from build123d import *

# Parameters (mm, degrees)
SKETCH1_R           = 7
SKETCH1_R_2         = 5.5
BOSS_EXTRUDE1_DEPTH = 7
SKETCH2_R           = 7
SKETCH2_R_2         = 4
BOSS_EXTRUDE2_DEPTH = 7
BOSS_EXTRUDE3_DEPTH = 4.5
CUT_EXTRUDE2_DEPTH  = 2


with BuildPart() as part:
    # Sketch1 → Boss-Extrude1 (new body, symmetric)
    with BuildSketch(Plane.XY):
        Circle(SKETCH1_R)
        Circle(SKETCH1_R_2, mode=Mode.SUBTRACT)
    extrude(amount=BOSS_EXTRUDE1_DEPTH, both=True)



with BuildPart() as body_2:
    # Sketch2 → Boss-Extrude2 (new body, symmetric)
    with BuildSketch(Plane.XY):
        with Locations((0, 80)):
            Circle(SKETCH2_R)
        with Locations((0, 80)):
            Circle(SKETCH2_R_2, mode=Mode.SUBTRACT)
    extrude(amount=BOSS_EXTRUDE2_DEPTH, both=True)


with BuildPart() as part_1:
    add(part.part)

    add(body_2.part)  # Boss-Extrude3 merges body 2
    # Sketch3 → Boss-Extrude3 (add, symmetric)
    with BuildSketch(Plane.XY):
        with BuildLine():
            Line((-5.25, 75.369935206), (-5.25, 4.630064794))
            ThreePointArc((-5.25, 4.630064794), (0, 7), (5.25, 4.630064794))
            Line((5.25, 4.630064794), (5.25, 75.369935206))
            ThreePointArc((5.25, 75.369935206), (0, 73), (-5.25, 75.369935206))
        make_face()
    extrude(amount=BOSS_EXTRUDE3_DEPTH, both=True)

    # Sketch4 → Cut-Extrude2 (cut)
    with BuildSketch(Plane.XY.offset(4.5)):
        with BuildLine():
            ThreePointArc((-3, 67.154767421), (-2.650443636, 67.914321947), (-1.846153846, 68.142862235))
            ThreePointArc((-1.846153846, 68.142862235), (0, 68), (1.846153846, 68.142862235))
            ThreePointArc((1.846153846, 68.142862235), (2.650443636, 67.914321947), (3, 67.154767421))
            Line((3, 67.154767421), (3, 12.845232579))
            ThreePointArc((3, 12.845232579), (2.650443636, 12.085678053), (1.846153846, 11.857137765))
            ThreePointArc((1.846153846, 11.857137765), (0, 12), (-1.846153846, 11.857137765))
            ThreePointArc((-1.846153846, 11.857137765), (-2.650443636, 12.085678053), (-3, 12.845232579))
            Line((-3, 12.845232579), (-3, 67.154767421))
        make_face()
    cut_extrude2 = extrude(amount=-CUT_EXTRUDE2_DEPTH, mode=Mode.SUBTRACT)

    # Mirror1: Cut-Extrude2 across plane
    add(cut_extrude2.mirror(Plane.XY), mode=Mode.SUBTRACT)


solid = part_1.part
The listing builds one solid part. Answer for the finished solid, in the listing's coordinates (mm). A direction names the side the tool comes from. Round coordinates to 2 decimals unless told otherwise and drop trailing zeros. Order: outer loops, then holes, each group sorted by start corner. A loop starts at its lowest first (then second) coordinate and runs counter-clockwise, first axis right, second up. Notation, with made-up numbers: (-27.75, -3) - (-14.75, -3) arc R21 ccw to (-14.75, 31) - close; hole circle Ø8 at (54.5, -31.75). An arc over 180 degrees is marked (long way). Write item = value, one per line. Start each with the question number.
1) Section A-A, the plane x = 0 is taken. Write down the section's boundary in (y, z).
2) Given pin 1 (3 mm diameter, centred on x = 2.5, y = 34.5, fed in from +Z); pin 2 (2 mm diameter, centred on x = -1.5, y = 47, fed in from +Z); pin 3 (0.6 mm diameter, centred on y = 44.5, z = 3.5, fed in from +X), each flat-ended and moving along its own axis, determine where each tip first touches the part or whether it passes through.
3) Section D-D, the plane y = 27 is taken. Write down the section's boundary in (x, z), plus the area to 3 significant figures.
4) Straight lines are drawn through the part: L1, parallel to Y at x = 0, z = -2; L2, parallel to X at y = 25, z = -2.75; L3, parallel to Y at x = 1.25, z = 3.5. For each, find the intervals that lie inside material, in ascending order.
5) For faces 1 (the cylindrical face through (0, 68, 4)), 2 (the flat face through (5.25, 40, 0)), 3 (the cylindrical face through (0, 68, -4)), 4 (the flat face through (-5.25, 40, 0)), determine the directions among +Z, -Z, +X, -X, +Y, -Y from which every point of the face is accessible in a straight line to the end or side of a thin tool.
6) Section B-B, the plane y = 80 is taken. Write down the section's boundary in (x, z), plus the area to 3 significant figures.
7) Section C-C, the plane z = -5.5 is taken. Write down the section's boundary in (x, y), plus the area to 3 significant figures.
Results list:
q1.outline = (-7, -7) - (-5.5, -7) - (-5.5, 7) - (-7, 7) - close; (5.5, -7) - (7, -7) - (7, -4.5) - (12, -4.5) - (12, -2.5) - (68, -2.5) - (68, -4.5) - (73, -4.5) - (73, -7) - (76, -7) - (76, 7) - (73, 7) - (73, 4.5) - (68, 4.5) - (68, 2.5) - (12, 2.5) - (12, 4.5) - (7, 4.5) - (7, 7) - (5.5, 7) - close; (84, -7) - (87, -7) - (87, 7) - (84, 7) - close
q2.pin_1 = 4.5
q2.pin_2 = 2.5
q2.pin_3 = 5.25
q3.outline = (-5.25, -4.5) - (-3, -4.5) - (-3, -2.5) - (3, -2.5) - (3, -4.5) - (5.25, -4.5) - (5.25, 4.5) - (3, 4.5) - (3, 2.5) - (-3, 2.5) - (-3, 4.5) - (-5.25, 4.5) - close
q3.area = 70.5 mm^2
q4.L1 = -7 to -5.5, 5.5 to 76, 84 to 87
q4.L2 = -5.25 to -3, 3 to 5.25
q4.L3 = -6.89 to -5.36, 5.36 to 11.93, 68.07 to 76.2, 83.8 to 86.89
q5.face_1 = +Z
q5.face_2 = +Z, -Z, +X
q5.face_3 = -Z
q5.face_4 = +Z, -Z, -X
q6.outline = (-7, -7) - (-4, -7) - (-4, 7) - (-7, 7) - close; (4, -7) - (7, -7) - (7, 7) - (4, 7) - close
q6.area = 84.0 mm^2
q7.outline = circle Ø14 at (0, 0); circle Ø14 at (0, 80); hole circle Ø11 at (0, 0); hole circle Ø8 at (0, 80)
q7.area = 163 mm^2
